from build123d import *

# Parameters (mm, degrees)
SKETCH1_W                      = 450
SKETCH1_H                      = 45
BOSS_EXTRUDE1_DEPTH            = 2
TERMINAL_12P_CUTOUT_DEPTH      = 227.131046077
TERMINAL_12P_CUTOUT_DEPTH_BACK = 227.131046077
SK_TERMINAL_12P_CUTOUT_R       = 1.625
SK_TERMINAL_12P_CUTOUT_W       = 56.92
SK_TERMINAL_12P_CUTOUT_H       = 10.9
SK_TERMINAL_12P_CUTOUT_W_2     = 34.06
SKETCH2_R                      = 2.5
CUT_EXTRUDE1_DEPTH             = 227.131046077
SKETCH3_R                      = 1.5
SKETCH3_R_2                    = 10
CUT_EXTRUDE2_DEPTH             = 10


with BuildPart() as part:
    # Sketch1 → Boss-Extrude1 (new body)
    with BuildSketch(Plane.XY):
        Rectangle(SKETCH1_W, SKETCH1_H)
    extrude(amount=BOSS_EXTRUDE1_DEPTH)

    # SK Terminal 12P cutout → Terminal 12P cutout (cut, two sides: drawn at the far end of the back side and taken through both)
    with BuildSketch(Plane.XY.offset(-TERMINAL_12P_CUTOUT_DEPTH_BACK)):
        with Locations((7.5, -8.35)):
            Circle(SK_TERMINAL_12P_CUTOUT_R)
        with Locations((69.67, -8.35)):
            Circle(SK_TERMINAL_12P_CUTOUT_R)
        with Locations((-46.81, -8.35)):
            Circle(SK_TERMINAL_12P_CUTOUT_R)
        with Locations((-7.5, -8.35)):
            Circle(SK_TERMINAL_12P_CUTOUT_R)
        with Locations((38.585, -8.95)):
            Rectangle(SK_TERMINAL_12P_CUTOUT_W, SK_TERMINAL_12P_CUTOUT_H)
        with Locations((-27.155, -8.95)):
            Rectangle(SK_TERMINAL_12P_CUTOUT_W_2, SK_TERMINAL_12P_CUTOUT_H)
    extrude(amount=TERMINAL_12P_CUTOUT_DEPTH + TERMINAL_12P_CUTOUT_DEPTH_BACK, mode=Mode.SUBTRACT)

    # Sketch2 → Cut-Extrude1 (cut, through all)
    with BuildSketch(Plane.XY.offset(2)):
        with Locations((-215, 0)):
            Circle(SKETCH2_R)
        with Locations((215, 0)):
            Circle(SKETCH2_R)
        with Locations((-194, 12.495407459)):
            Circle(SKETCH2_R)
        with Locations((194, 12.495407459)):
            Circle(SKETCH2_R)
        with Locations((0, 12.5)):
            Circle(SKETCH2_R)
    extrude(amount=-CUT_EXTRUDE1_DEPTH, mode=Mode.SUBTRACT)

    # Sketch3 → Cut-Extrude2 (cut)
    with BuildSketch(Plane.XY.offset(2)):
        with Locations((150, -8.55)):
            Circle(SKETCH3_R)
        with Locations((175, -8.55)):
            Circle(SKETCH3_R)
        with Locations((80, -8.55)):
            Circle(SKETCH3_R)
        with Locations((105, -8.55)):
            Circle(SKETCH3_R)
        with Locations((194, -8.55)):
            Circle(SKETCH3_R_2)
        with Locations((-194, -8.55)):
            Circle(SKETCH3_R_2)
        with BuildLine():
            Line((168.375, -14.4), (154.1, -14.4))
            ThreePointArc((154.1, -14.4), (153.392893219, -14.107106781), (153.1, -13.4))
            Line((153.1, -13.4), (153.1, -3.7))
            ThreePointArc((153.1, -3.7), (153.451471863, -2.851471863), (154.3, -2.5))
            Line((154.3, -2.5), (168.175, -2.5))
            ThreePointArc((168.175, -2.5), (170.80897276, -3.59102724), (171.9, -6.225))
            Line((171.9, -6.225), (171.9, -10.875))
            ThreePointArc((171.9, -10.875), (170.867551404, -13.367551404), (168.375, -14.4))
        make_face()
        with BuildLine():
            Line((98.375, -14.4), (84.1, -14.4))
            ThreePointArc((84.1, -14.4), (83.392893219, -14.107106781), (83.1, -13.4))
            Line((83.1, -13.4), (83.1, -3.7))
            ThreePointArc((83.1, -3.7), (83.451471863, -2.851471863), (84.3, -2.5))
            Line((84.3, -2.5), (98.175, -2.5))
            ThreePointArc((98.175, -2.5), (100.80897276, -3.59102724), (101.9, -6.225))
            Line((101.9, -6.225), (101.9, -10.875))
            ThreePointArc((101.9, -10.875), (100.867551404, -13.367551404), (98.375, -14.4))
        make_face()
    extrude(amount=-CUT_EXTRUDE2_DEPTH, mode=Mode.SUBTRACT)


solid = part.part
The listing builds one solid part. Answer for the finished solid, in the listing's coordinates (mm). Give positions to 0.01 mm unless a question says otherwise; leave off trailing zeros.
Item 1: Determine the mould class of faces 1 (the flat face through (-3, 0, 0)), 2 (the cylindrical face through (-184.763, -12.38, 1.014)), 3 (the cylindrical face through (203.237, -12.38, 1.014)) for opening direction Y: released by +Y, released by -Y, zero draft, split by the parting line, or undercut.
Item 2: Section A-A, the plane z = 1.6 is taken. Count the separate pieces of the cut face and the enclosed holes in it, plus the area to 3 significant figures.
Item 3: Find the intervals of material crossed by line 1 along Y through (x, z) = (69.67, 1.15) (3 decimals); line 2 along Y through (x, z) = (28, 0.6); line 3 along X through (y, z) = (-17.5, 1.15), in increasing order.
Completed:
1. face 1: zero draft
1. face 2: undercut
1. face 3: undercut
2. separate pieces: 1
2. enclosed holes: 19
2. area: 18,000 mm2
3. line 1: y = -22.5 to -9.975, -6.725 to 22.5
3. line 2: y = -22.5 to -14.4, -3.5 to 22.5
3. line 3: x = -225 to -198.46, -189.54 to 189.54, 198.46 to 225
